Verification items for this drawing (mm, ordinates from the low corner). A direction names the side the tool comes from. Give positions to 0.01 mm unless a question says otherwise; leave off trailing zeros. Loops run counter-clockwise (first coordinate to the right, second up) from the corner with the lowest first, then second, coordinate; pieces in that order, holes last. Notation, with made-up numbers: (61, 42.5) -> (81, 42.5) arc R14 ccw to (81, 68.5) -> close; hole circle Ø8 at (-1.5, -23.5). An arc over 180 degrees is marked (long way). Write item = value, one per line.
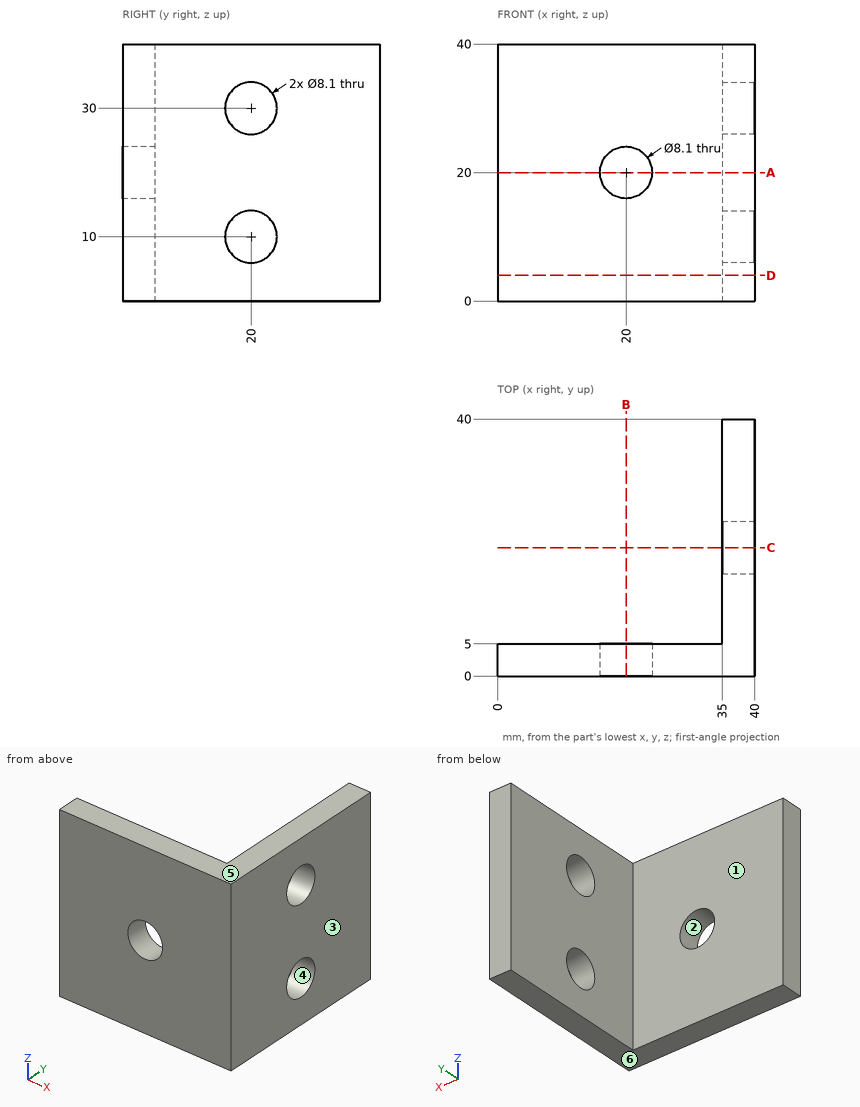
Item 1: Tool access check on the marked faces 1 and 2. Record the directions out of +Z, -Z, +X, -X, +Y, -Y that give a thin tool (end or side, any length) a straight path to the whole face; none if there is none.
Answer:
face_1 = +Z, -Z, -X, +Y
face_2 = +Y, -Y
Item 2: Thickness scan on L1, parallel to Y at x = 37.25, z = 30; L2, parallel to Y at x = 11, z = 22. Record the ranges inside material, lowest first. Write a range as [from, to].
Answer:
L1 = [0, 15.95], [24.05, 40]
L2 = [0, 5]
Item 3: Section check B-B, the plane x = 20. Record the cut outline in (y, z), plus the area to 4 significant figures.
Answer:
outline = (0, 0) -> (5, 0) -> (5, 15.95) -> (0, 15.95) -> close; (0, 24.05) -> (5, 24.05) -> (5, 40) -> (0, 40) -> close
area = 159.5 mm^2
Item 4: Section check D-D, the plane z = 4. Record the cut outline in (x, y).
Answer:
outline = (0, 0) -> (40, 0) -> (40, 40) -> (35, 40) -> (35, 5) -> (0, 5) -> close
Item 5: Section check A-A, the plane z = 20. Record the cut outline in (x, y), plus the area to 4 significant figures.
Answer:
outline = (0, 0) -> (15.95, 0) -> (15.95, 5) -> (0, 5) -> close; (24.05, 0) -> (40, 0) -> (40, 40) -> (35, 40) -> (35, 5) -> (24.05, 5) -> close
area = 334.5 mm^2
Item 6: Section check C-C, the plane y = 20. Record the cut outline in (x, z).
Answer:
outline = (35, 0) -> (40, 0) -> (40, 5.95) -> (35, 5.95) -> close; (35, 14.05) -> (40, 14.05) -> (40, 25.95) -> (35, 25.95) -> close; (35, 34.05) -> (40, 34.05) -> (40, 40) -> (35, 40) -> close
Item 7: Gauge pin test, flat ends, axial feed: pin 1 (10.5 mm diameter, centred on y = 20, z = 30, fed in from -X); pin 2 (10 mm diameter, centred on x = 8, z = 36, fed in from +Y); pin 3 (5 mm diameter, centred on x = 20, z = 20, fed in from +Y). Record the tip position at first contact, or that the pin passes through.
Answer:
pin_1 = 35
pin_2 = 5
pin_3 = through
Item 8: Draft check along Z on the marked faces 3, 4, 5 and 6. Enter one of: +Z half, -Z half, draft (parallel to the pull), parting line (faces both ways), or undercut.
Answer:
face_3 = draft
face_4 = undercut
face_5 = +Z half
face_6 = -Z half
